The listing builds one solid part. Answer for the finished solid, in the listing's coordinates (mm). A direction names the side the tool comes from. Coordinates: 2 decimals unless noted, no trailing zeros. Order: outer loops, then holes, each group sorted by start corner. A loop starts at its lowest first (then second) coordinate and runs counter-clockwise, first axis right, second up. Notation, with made-up numbers: (-4.5, -10) - (53.5, -10) arc R23 ccw to (53.5, 12) - close; hole circle Ø7 at (-18, 69.25). An arc over 180 degrees is marked (long way). Use a Markdown table: item, result. Add a question column.
Item 1: The part is cut by section B-B, the plane z = 0. Give the vertices of the cut face in (x, y).
Item 2: For faces 1 (the flat face through (1, 1.4, 1)), 2 (the flat face through (-2.6, 1.17, 0)), determine the directions among +Z, -Z, +X, -X, +Y, -Y from which every point of the face is accessible in a straight line to the end or side of a thin tool.
Item 3: Find the intervals of material crossed by line 1 along X through (y, z) = (1.2, 0); line 2 along Y through (x, z) = (-2.75, 2); line 3 along Z through (x, y) = (-1.25, -1.15), in increasing order.
Item 4: The part is cut by section A-A, the plane x = 0. Give the vertices of the cut face in (y, z).
Item 5: The part is cut by section C-C, the plane y = -0.85. Give the vertices of the cut face in (x, z), then the cut area to 3 significant figures.
Item 6: Flat-ended cylindrical pins translate along their axes: P1, Ø1.5, axis at x = 0, z = 0, coming from the +Y side; P2, Ø0.8, axis at x = -4, z = 2, coming from the +Y side. Find the tip coordinate at first contact, or state that the pin passes through.
Item 7: The part is cut by section D-D, the plane y = 0.6. Give the vertices of the cut face in (x, z), then the cut area to 3 significant figures.
from build123d import *

# Parameters (mm, degrees)
SKETCH1_W               = 6.7
SKETCH1_H               = 6.7
BOSS_EXTRUDE1_DEPTH     = 1.4
SKETCH2_W               = 0.4
SKETCH2_H               = 0.2
BOSS_EXTRUDE2_DEPTH     = 0.8
LPATTERN1_COUNT         = 3
LPATTERN1_PITCH         = 1.27
LPATTERN1_COL_COUNT     = 2
LPATTERN1_COL_PITCH     = 1.27
MIRROR1_COPY_1_SKETCH_W = 0.4
MIRROR1_COPY_1_SKETCH_H = 0.2
MIRROR1_COPY_1_DEPTH    = 0.8
MIRROR1_COPY_2_SKETCH_W = 0.4
MIRROR1_COPY_2_SKETCH_H = 0.2
MIRROR1_COPY_2_DEPTH    = 0.8
MIRROR1_COPY_3_SKETCH_W = 0.4
MIRROR1_COPY_3_SKETCH_H = 0.2
MIRROR1_COPY_3_DEPTH    = 0.8
SKETCH3_W               = 0.8
SKETCH3_H               = 0.2
BOSS_EXTRUDE3_DEPTH     = 0.8
FILLET1_R               = 0.55
DRAFT1_ANGLE            = 2.5
SKETCH4_R               = 1.25
CUT_EXTRUDE1_DEPTH      = 0.55
SKETCH5_R               = 2.4
CUT_EXTRUDE2_DEPTH      = 0.23


with BuildPart() as part:
    # Sketch1 → Boss-Extrude1 (new, symmetric)
    with BuildSketch(Plane(origin=(0, 0, 0), x_dir=(1, 0, 0), z_dir=(0, 1, 0))):
        Rectangle(SKETCH1_W, SKETCH1_H)
    extrude(amount=BOSS_EXTRUDE1_DEPTH, both=True)

    # Sketch2 → Boss-Extrude2 (add)
    with BuildSketch(Plane(origin=(3.35, 0, 0), x_dir=(0, 0, -1), z_dir=(1, 0, 0))):
        with Locations((-0.635, -1.3)):
            Rectangle(SKETCH2_W, SKETCH2_H)
    boss_extrude2 = extrude(amount=BOSS_EXTRUDE2_DEPTH)

    # LPattern1: Boss-Extrude2 ×3
    with Locations(*[(0, 0, -i * LPATTERN1_PITCH) for i in range(1, LPATTERN1_COUNT)]):
        add(boss_extrude2)

    # LPattern1 col: Boss-Extrude2 ×2
    with Locations(*[(0, 0, i * LPATTERN1_COL_PITCH) for i in range(1, LPATTERN1_COL_COUNT)]):
        add(boss_extrude2)

    # Mirror1: Boss-Extrude2 across plane
    add(boss_extrude2.mirror(Plane(origin=(0, 0, 0), x_dir=(0, 0, 1), z_dir=(1, 0, 0))))

    # Mirror1 copy 1 sketch → Mirror1 copy 1 (add)
    with BuildSketch(Plane(origin=(-3.35, 0, -1.27), x_dir=(0, 0, -1), z_dir=(-1, 0, 0))):
        with Locations((-0.635, 1.3)):
            Rectangle(MIRROR1_COPY_1_SKETCH_W, MIRROR1_COPY_1_SKETCH_H)
    extrude(amount=MIRROR1_COPY_1_DEPTH)

    # Mirror1 copy 2 sketch → Mirror1 copy 2 (add)
    with BuildSketch(Plane(origin=(-3.35, 0, -2.54), x_dir=(0, 0, -1), z_dir=(-1, 0, 0))):
        with Locations((-0.635, 1.3)):
            Rectangle(MIRROR1_COPY_2_SKETCH_W, MIRROR1_COPY_2_SKETCH_H)
    extrude(amount=MIRROR1_COPY_2_DEPTH)

    # Mirror1 copy 3 sketch → Mirror1 copy 3 (add)
    with BuildSketch(Plane(origin=(-3.35, 0, 1.27), x_dir=(0, 0, -1), z_dir=(-1, 0, 0))):
        with Locations((-0.635, 1.3)):
            Rectangle(MIRROR1_COPY_3_SKETCH_W, MIRROR1_COPY_3_SKETCH_H)
    extrude(amount=MIRROR1_COPY_3_DEPTH)

    # Sketch3 → Boss-Extrude3 (add)
    with BuildSketch(Plane.ZY.offset(3.35)):
        with Locations((1.905, -1.3)):
            Rectangle(SKETCH3_W, SKETCH3_H)
    extrude(amount=BOSS_EXTRUDE3_DEPTH)

    # Fillet1
    fillet1_edges = [part.edges().sort_by_distance(p)[0] for p in [
        (3.35, 0, -3.35),
        (3.35, 0, 3.35),
        (-3.35, 0, 3.35),
        (-3.35, 0, -3.35),
    ]]
    fillet(fillet1_edges, radius=FILLET1_R)

    # Draft1
    draft1_faces = [part.faces().sort_by_distance(p)[0] for p in [
        (3.18890873, 0, 3.18890873),
        (3.35, 0.027083333, 0),
        (3.18890873, 0, -3.18890873),
        (-3.18890873, 0, -3.18890873),
        (-3.18890873, 0, 3.18890873),
        (0, 0, 3.35),
        (-3.35, 0.034031414, -0.009973822),
        (0, 0, -3.35),
    ]]
    draft(draft1_faces, Plane.ZX.offset(1.4), DRAFT1_ANGLE)

    # Sketch4 → Cut-Extrude1 (cut)
    with BuildSketch(Plane(origin=(0, 1.4, 0), x_dir=(1, 0, 0), z_dir=(0, 1, 0))):
        with Locations(Location((0, 0, 0), (0, 0, 270))):
            Circle(SKETCH4_R)
    extrude(amount=-CUT_EXTRUDE1_DEPTH, mode=Mode.SUBTRACT)

    # Sketch5 → Cut-Extrude2 (cut)
    with BuildSketch(Plane(origin=(0, 1.4, 0), x_dir=(1, 0, 0), z_dir=(0, 1, 0))):
        with BuildLine():
            Line((-2.34, -2.89), (2.34, -2.89))
            ThreePointArc((2.34, -2.89), (2.72890873, -2.72890873), (2.89, -2.34))
            Line((2.89, -2.34), (2.89, 2.34))
            ThreePointArc((2.89, 2.34), (2.72890873, 2.72890873), (2.34, 2.89))
            Line((2.34, 2.89), (-2.34, 2.89))
            ThreePointArc((-2.34, 2.89), (-2.72890873, 2.72890873), (-2.89, 2.34))
            Line((-2.89, 2.34), (-2.89, -2.34))
            ThreePointArc((-2.89, -2.34), (-2.72890873, -2.72890873), (-2.34, -2.89))
        make_face()
        with Locations(Location((0, 0, 0), (0, 0, 270))):
            Circle(SKETCH5_R, mode=Mode.SUBTRACT)
    extrude(amount=-CUT_EXTRUDE2_DEPTH, mode=Mode.SUBTRACT)


solid = part.part
Solution:
| question | item | result |
|---|---|---|
| 1 | outline | (-3.47, -1.4) - (3.47, -1.4) - (3.35, 1.4) - (2.89, 1.4) - (2.89, 1.17) - (2.4, 1.17) - (2.4, 1.4) - (1.25, 1.4) - (1.25, 0.85) - (-1.25, 0.85) - (-1.25, 1.4) - (-2.4, 1.4) - (-2.4, 1.17) - (-2.89, 1.17) - (-2.89, 1.4) - (-3.35, 1.4) - close |
| 2 | face 1 | +Z, -Z, +X, -X, +Y |
| 2 | face 2 | +Y |
| 3 | line 1 | x = -3.36 to -2.89, -2.4 to -1.25, 1.25 to 2.4, 2.89 to 3.36 |
| 3 | line 2 | y = -1.4 to 1.17 |
| 3 | line 3 | z = -3.46 to 3.46 |
| 4 | outline | (-1.4, -3.47) - (1.4, -3.35) - (1.4, -2.89) - (1.17, -2.89) - (1.17, -2.4) - (1.4, -2.4) - (1.4, -1.25) - (0.85, -1.25) - (0.85, 1.25) - (1.4, 1.25) - (1.4, 2.4) - (1.17, 2.4) - (1.17, 2.89) - (1.4, 2.89) - (1.4, 3.35) - (-1.4, 3.47) - close |
| 5 | outline | (-3.45, -2.8) arc R0.65 ccw to (-2.8, -3.45) - (2.8, -3.45) arc R0.65 ccw to (3.45, -2.8) - (3.45, 2.8) arc R0.65 ccw to (2.8, 3.45) - (-2.8, 3.45) arc R0.65 ccw to (-3.45, 2.8) - close |
| 5 | area | 47.2 mm2 |
| 6 | P1 | stops at y = 0.85 |
| 6 | P2 | stops at y = -1.2 |
| 7 | outline | (-3.38, -2.8) arc R0.58 ccw to (-2.8, -3.38) - (2.8, -3.38) arc R0.58 ccw to (3.38, -2.8) - (3.38, 2.8) arc R0.58 ccw to (2.8, 3.38) - (-2.8, 3.38) arc R0.58 ccw to (-3.38, 2.8) - close |
| 7 | area | 45.5 mm2 |
